Could you check a few things on this model? Use its own coordinates, in mm. A direction names the side the tool comes from. Round coordinates to 2 decimals unless told otherwise and drop trailing zeros. Order: outer loops, then holes, each group sorted by start corner. A loop starts at its lowest first (then second) coordinate and runs counter-clockwise, first axis right, second up. Notation, with made-up numbers: (16, 87) -> (47, 87) arc R14 ccw to (47, 101) -> close; hole circle Ø6 at (12.5, 70.5). An arc over 180 degrees is marked (long way). Put each result on its own line as item: value. Start each with the question number.
from build123d import *

# Parameters (mm, degrees)
SKETCH_1_R      = 5
SKETCH_1_R_2    = 2.1
SKETCH_1_R_3    = 6.75
SKETCH_1_R_4    = 1.6
EXTRUDE_1_DEPTH = 3
FILLET_1_R      = 10
FILLET_2_R      = 10


with BuildPart() as part:
    # 草图1 → 凸台-拉伸1 (new body)
    with BuildSketch(Plane.XY):
        with BuildLine():
            Line((12.419223494, -15.676826458), (153.603692908, -23.133474126))
            ThreePointArc((153.603692908, -23.133474126), (157.711237696, -22.783135564), (161.568286957, -21.32785817))
            Line((161.568286957, -21.32785817), (192.671157578, -4.391169028))
            ThreePointArc((192.671157578, -4.391169028), (195.155704471, 1.10792866), (190.538680801, 4.993303941))
            Line((190.538680801, 4.993303941), (155.185935535, 6.824771956))
            Line((155.185935535, 6.824771956), (14.001466121, 14.281419623))
            ThreePointArc((14.001466121, 14.281419623), (-19.972164054, 1.054828418), (12.419223494, -15.676826458))
        make_face()
        with Locations((154.394814221, -8.154351085)):
            Circle(SKETCH_1_R, mode=Mode.SUBTRACT)
        with Locations((190.28, 0)):
            Circle(SKETCH_1_R_2, mode=Mode.SUBTRACT)
        Circle(SKETCH_1_R_3, mode=Mode.SUBTRACT)
        with Locations((0, 9.5)):
            Circle(SKETCH_1_R_4, mode=Mode.SUBTRACT)
        with Locations((0, 16)):
            Circle(SKETCH_1_R_4, mode=Mode.SUBTRACT)
        with Locations((8.227241336, -4.75)):
            Circle(SKETCH_1_R_4, mode=Mode.SUBTRACT)
        with Locations((-8.227241336, -4.75)):
            Circle(SKETCH_1_R_4, mode=Mode.SUBTRACT)
        with Locations((13.856406461, -8)):
            Circle(SKETCH_1_R_4, mode=Mode.SUBTRACT)
        with Locations((-13.856406461, -8)):
            Circle(SKETCH_1_R_4, mode=Mode.SUBTRACT)
    extrude(amount=EXTRUDE_1_DEPTH)

    # 圆角1
    fillet_1_edges = [part.edges().sort_by_distance(p)[0] for p in [
        (14.001466121, 14.281419623, 1.5),
    ]]
    fillet(fillet_1_edges, radius=FILLET_1_R)

    # 圆角2
    fillet_2_edges = [part.edges().sort_by_distance(p)[0] for p in [
        (12.419223494, -15.676826458, 1.5),
    ]]
    fillet(fillet_2_edges, radius=FILLET_2_R)


solid = part.part
1. I need wall thicknesses on L1, parallel to Y at x = 0, z = 1; L2, parallel to Y at x = 150.5, z = 2.5; L3, parallel to Y at x = -7, z = 1.35 (3 decimals). Which ranges of each line are inside material? Lowest first, please.
2. Which directions (+Z, -Z, +X, -X, +Y, -Y) give clear straight access to the entire face, cutting with the end or side of a thin tool? Please do faces 1 (the face through (188.18, 0.09, 1.48)), 2 (the face through (83.721, -19.443, 1.479)).
3. For pin 1 Ø2.5 at (x, y) = (0, 9.5) entering from -Z, with a flat end and sliding along its axis, tell me the tip position at first contact or that it passes through.
4. If we section it at A-A, the plane z = 0.7: Count the separate pieces of the cut face and the enclosed holes in it, then the cut area to 3 significant figures.
5. Thinking about a two-plate mould opening in X: for faces 3 (the face through (-1.46, -6.59, 1.48)), 4 (the face through (86, -6, 3)), 5 (the face through (176.9, -12.98, 1.48)), which applies, +X half, -X half, draft (parallel to the pull), parting line (faces both ways), or undercut?
6. If we section it at B-B, the plane x = 144: Please give me the cut outline in (y, z).
Results below:
1. L1: -20 to -6.75, 6.75 to 7.9, 11.1 to 14.4, 17.6 to 20
1. L2: -22.97 to -11.29, -5.02 to 7.07
1. L3: -18.735 to -5.777, -3.723 to 18.735
2. face 1: +Z, -Z
2. face 2: +Z, -Z, -Y
3. pin 1: through
4. separate pieces: 1
4. enclosed holes: 9
4. area: 5,880 mm2
5. face 3: undercut
5. face 4: draft
5. face 5: +X half
6. outline: (-22.63, 0) -> (7.42, 0) -> (7.42, 3) -> (-22.63, 3) -> close
